from build123d import *

# Parameters (mm, degrees)
F3_SIZE = 2
F4_R    = 3.5


with BuildPart() as f2:
    # F1 (on Front) → F2 (revolve)
    with BuildSketch(Plane.XZ):
        Polygon((0, 46), (0, 31.54), (6.4, 31.54), (6.4, 34.95), (6.4, 38.45), (9.9, 38.45), (13.5, 38.45), (13.5, 46), align=None)
    revolve(axis=Axis((6.796166, 0, 0), (1, 0, 0)))

    # F3
    f3_edges = [f2.edges().sort_by_distance(p)[0] for p in [
        (0, 0, -46),
    ]]
    chamfer(f3_edges, length=F3_SIZE)

    # F4
    f4_edges = [f2.edges().sort_by_distance(p)[0] for p in [
        (6.4, 0, -38.45),
    ]]
    fillet(f4_edges, radius=F4_R)


solid = f2.part
Source: CAD feature listing. Evaluate the final solid. Frame: model axes, mm. A direction names the side the tool comes from. Give positions to 0.01 mm unless a question says otherwise; leave off trailing zeros. Write each loop counter-clockwise with the first axis right and the second up, starting at its lowest first coordinate (ties: lowest second). Pieces come first, ordered by that corner, then holes. Notation, with made-up numbers: M -31.5,62 L 0.5,62 A22 ccw 0.5,85 Z; hole C 9,64.25 d9. An arc over 180 degrees is marked long. Answer as a JSON object with one key per item and string values.
Q1. Cut plane A-A, the plane z = 0. Return the cut outline in (x, y).
Geometry check:
{"outline": "M 0,-44 L 2,-46 L 13.5,-46 L 13.5,-38.45 L 9.9,-38.45 A3.5 cw 6.4,-34.95 L 6.4,-31.54 L 0,-31.54 Z; M 0,31.54 L 6.4,31.54 L 6.4,34.95 A3.5 cw 9.9,38.45 L 13.5,38.45 L 13.5,46 L 2,46 L 0,44 Z"}
Q2. Contact query for flat-ended pins moving along their axis: P1, Ø10, axis at y = -17.5, z = -26, coming from the -X side; P2, Ø8, axis at x = 10, z = -2.5, coming from the +Y side; P3, Ø6, axis at x = 10.5, y = -28, coming from the -Z side. Output: stop coordinate, or through.
Geometry check:
{"P1": "stops at x = 0", "P2": "stops at y = 46", "P3": "stops at z = -38.61"}
Q3. Mould query, pull axis Z, two halves, no side actions, for faces 3 (the face through (13.5, 37.3, 10.4)), 4 (the face through (3.245, -21.316, -23.246)), 5 (the face through (7.67, -45.61, -5.99)). Classes: +Z half, -Z half, draft (parallel to the pull), parting line (faces both ways), or undercut.
Geometry check:
{"face 3": "draft", "face 4": "undercut", "face 5": "parting line"}
Q4. Ray query, line 1 along Z through (x, y) = (2.25, 0); line 2 along Z through (x, y) = (11.45, 0). Return the intervals inside material, ascending.
Geometry check:
{"line 1": "z = -46 to -31.54, 31.54 to 46", "line 2": "z = -46 to -38.45, 38.45 to 46"}
Q5. Cut plane D-D, the plane x = 12.25. Return the cut outline in (y, z).
Geometry check:
{"outline": "C 0,0 d92; hole C 0,0 d76.9"}
Q6. Access query for faces 1 (the face through (11.725, -11.549, 36.674)), 2 (the face through (0.13, 43.08, -9.57)). Directions: +Z, -Z, +X, -X, +Y, -Y. A direction counts if a zero-diameter tool reaches every point of the face in a straight line with its end or side. Return the directions, or none.
Geometry check:
{"face 1": "+X", "face 2": "-X"}
Q7. Cut plane C-C, the plane x = 5. Return the cut outline in (y, z), then the cut area to 3 significant figures.
Geometry check:
{"outline": "C 0,0 d92; hole C 0,0 d63.08", "area": "3,520 mm^2"}
